Autodesk Inventor part; units mm, degrees
ref_plane "YZ Plane" through (0, 0, 0) normal (1, 0, 0) x (0, 1, 0)
ref_plane "XZ Plane" through (0, 0, 0) normal (0, 1, 0) x (-1, 0, 0)
ref_plane "XY Plane" through (0, 0, 0) normal (0, 0, 1) x (1, 0, 0)
sketch "Sketch2" plane through (0, 0, 0) normal (0, 1, 0) x (-1, 0, 0)
  line L0 (-89, 99) -> (89, 99)
  line L1 (89, 99) -> (89, -99)
  line L2 (89, -99) -> (-89, -99)
  line L3 (-89, -99) -> (-89, 99)
  line L4 (-89, 99) -> (89, -99) construction
  line L5 (89, 99) -> (-89, -99) construction
  line L6 (-89, 99) -> (89, 99)
  line L7 (89, 99) -> (89, -81)
  line L8 (89, -81) -> (-89, -81)
  line L9 (-89, -81) -> (-89, 99)
  line L10 (-4.5, 99) -> (-89, 99)
  line L11 (-89, 99) -> (-89, 43)
  line L12 (-89, 43) -> (-4.5, 43)
  line L13 (-4.5, 43) -> (-4.5, 99)
  line L14 (4.5, 99) -> (89, 99)
  line L15 (89, 99) -> (89, 43)
  line L16 (89, 43) -> (4.5, 43)
  line L17 (4.5, 43) -> (4.5, 99)
  line L18 (22.5, 77.5) -> (22.5, 66.5)
  line L19 (16.5, 66.5) -> (16.5, 77.5)
  line L20 (-22.5, 66.5) -> (-22.5, 77.5)
  line L21 (-16.5, 77.5) -> (-16.5, 66.5)
  line L22 (-22.5, 99) -> (-16.5, 99)
  line L23 (-16.5, 99) -> (-16.5, 43)
  line L24 (-16.5, 43) -> (-22.5, 43)
  line L25 (-22.5, 43) -> (-22.5, 99)
  line L26 (16.5, 99) -> (22.5, 99)
  line L27 (22.5, 99) -> (22.5, 43)
  line L28 (22.5, 43) -> (16.5, 43)
  line L29 (16.5, 43) -> (16.5, 99)
  line L30 (-89, 99) -> (89, 99)
  line L31 (89, 99) -> (89, 98)
  line L32 (89, 98) -> (-89, 98)
  line L33 (-89, 98) -> (-89, 99)
  line L34 (89, -81) -> (74, -81)
  line L35 (74, -81) -> (74, -65)
  line L36 (74, -65) -> (89, -65)
  line L37 (89, -65) -> (89, -81)
  line L38 (-89, -81) -> (-74, -81)
  line L39 (-74, -81) -> (-74, -65)
  line L40 (-74, -65) -> (-89, -65)
  line L41 (-89, -65) -> (-89, -81)
  line L42 (16.5, 98) -> (-16.5, 98)
  line L43 (-16.5, 98) -> (-16.5, 94)
  line L44 (-16.5, 94) -> (16.5, 94)
  line L45 (16.5, 94) -> (16.5, 98)
  point P0 (0, 0)
  point P1 (4.5, 99)
  point P2 (-4.5, 99)
  point P3 (-89, 43)
  point P4 (89, 43)
  point P5 (4.5, 98)
  point P6 (-4.5, 98)
  point P7 (-16.5, 98)
  point P8 (-22.5, 98)
  point P9 (22.5, 98)
  point P10 (16.5, 98)
  point P11 (-4.5, 94)
  point P12 (4.5, 94)
  point P13 (16.5, 94)
  dimension "d8" = 178
  dimension "d9" = 198
  dimension "d10" = 18
  dimension "d11" = 84.5
  dimension "d13" = 84.5
  dimension "d17" = 9
  dimension "d18" = 1
  dimension "d19" = 15
  dimension "d20" = 16
  dimension "d21" = 15
  dimension "d22" = 16
  dimension "d75" = 55
  dimension "d76" = 55
  dimension "d77" = 6
  dimension "d78" = 6
  dimension "d79" = 4
extrude "Extrusion2" add sketch "Sketch2" along normal blind 3 contours L32 L23 L21 L12 L25 L20 | L12 L13 L44 L17 L16 L1 L36 L35 L8 L39 L40 L3 | L32 L13 L44 L23 | L32 L17 L44 L13 | L32 L29 L44 L17 | L32 L27 L18 L16 L29 L19
fillet "Fillet1" radius 3 6 edges at (22.5, 1.5, 43) (-22.5, 1.5, 43) (-16.5, 1.5, 43) (-4.5, 1.5, 43) (4.5, 1.5, 43) (16.5, 1.5, 43)
fillet "Fillet2" radius 3 2 edges at (74, 1.5, -65) (-74, 1.5, -65)
fillet "Fillet3" radius 3 4 edges at (16.5, 1.5, 94) (4.5, 1.5, 94) (-4.5, 1.5, 94) (-16.5, 1.5, 94)
equation "\"d11\" = d13"
properties part number "base" material "Aluminum 6061"
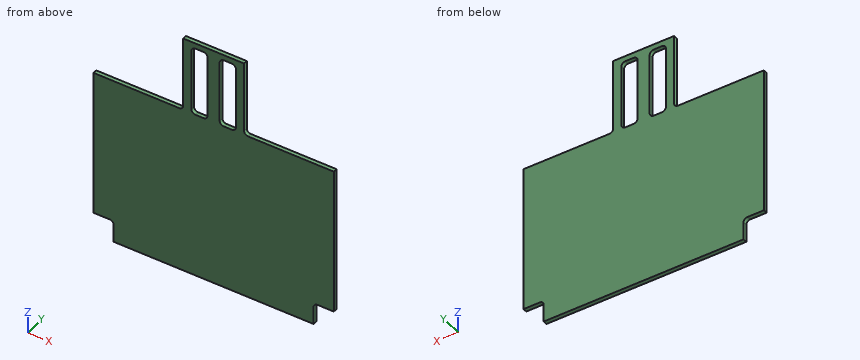
Check sheet for the modelled part. Datum: model origin and axes. Units: mm. Give positions to 0.01 mm unless a question says otherwise; leave off trailing zeros. Order: outer loops, then holes, each group sorted by start corner. A loop starts at its lowest first (then second) coordinate and runs counter-clockwise, first axis right, second up. Notation, with made-up numbers: M 20,66.25 L 79,66.25 A15 ccw 79,77.25 Z; hole C 55,19.25 d3. An arc over 180 degrees is marked long. Answer in a Markdown table with one row per item. Add a question column.
Q1. Sectioned sample at B-B, the plane y = 0.8. Count the separate pieces of the cut face and the enclosed holes in it, and give its area (3 significant figures).
Q2. Gauge pin test, flat ends, axial feed: pin 1 Ø0.9 at (x, y) = (-81.5, 2) entering from -Z; pin 2 Ø1.5 at (y, z) = (1.5, 72.5) entering from +X; pin 3 Ø12 at (x, z) = (71, -38.5) entering from -Y; pin 4 Ø1.5 at (y, z) = (2, 70) entering from -X. Record the tip position at first contact, or that the pin passes through.
Q3. Thickness scan on L1, parallel to X at y = 0.2, z = 62; L2, parallel to Z at x = -13, y = 1.85; L3, parallel to Z at x = 82, y = 2.9. Record the ranges inside material, lowest first.
Q4. Sectioned sample at A-A, the plane z = 61. Record the boundary of the cut face in (x, y).
Q5. Sectioned sample at C-C, the plane x = -52. Record the boundary of the cut face in (y, z), and give its area (3 significant figures).
Verdict:
| question | item | result |
|---|---|---|
| 1 | separate pieces | 1 |
| 1 | enclosed holes | 2 |
| 1 | area | 22,900 mm² |
| 2 | pin 1 | z = -65 |
| 2 | pin 2 | x = 22.5 |
| 2 | pin 3 | y = 0 |
| 2 | pin 4 | x = -22.5 |
| 3 | L1 | -22.5 to -16.5, -4.5 to 4.5, 16.5 to 22.5 |
| 3 | L2 | -81 to 43, 94 to 98 |
| 3 | L3 | -65 to 43 |
| 4 | outline | M -22.5,0 L -16.5,0 L -16.5,3 L -22.5,3 Z; M -4.5,0 L 4.5,0 L 4.5,3 L -4.5,3 Z; M 16.5,0 L 22.5,0 L 22.5,3 L 16.5,3 Z |
| 5 | outline | M 0,-81 L 3,-81 L 3,43 L 0,43 Z |
| 5 | area | 372 mm² |
